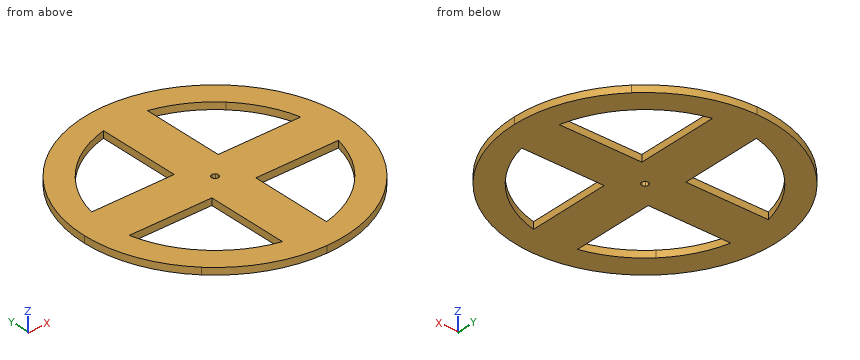
from build123d import *

# Parameters (mm, degrees)
F1_DEPTH = 3.175


with BuildPart() as f1:
    # F0 (on Top) → F1 (new body)
    with BuildSketch(Plane.XY):
        with BuildLine():
            Line((34.677494, 34.677494), (42.656217, 42.656217))
            ThreePointArc((42.656217, 42.656217), (23.085378, 55.733033), (0, 60.325))
            Line((0, 60.325), (0, 48.26))
            Line((0, 48.26), (10.16, 48.26))
            ThreePointArc((10.16, 48.26), (23.374034, 43.193116), (34.677494, 34.677494))
        make_face()
        with BuildLine():
            Line((48.26, 0), (60.325, 0))
            ThreePointArc((60.325, 0), (55.733033, 23.085378), (42.656217, 42.656217))
            Line((42.656217, 42.656217), (34.677494, 34.677494))
            ThreePointArc((34.677494, 34.677494), (43.193116, 23.374034), (48.26, 10.16))
            Line((48.26, 10.16), (48.26, 0))
        make_face()
        with BuildLine():
            Line((0, 48.26), (0, 60.325))
            ThreePointArc((0, 60.325), (-23.085378, 55.733033), (-42.656217, 42.656217))
            Line((-42.656217, 42.656217), (-34.677494, 34.677494))
            ThreePointArc((-34.677494, 34.677494), (-23.374034, 43.193116), (-10.16, 48.26))
            Line((-10.16, 48.26), (0, 48.26))
        make_face()
        with BuildLine():
            Line((-34.677494, 34.677494), (-42.656217, 42.656217))
            ThreePointArc((-42.656217, 42.656217), (-55.733033, 23.085378), (-60.325, 0))
            Line((-60.325, 0), (-48.26, 0))
            Line((-48.26, 0), (-48.26, 10.16))
            ThreePointArc((-48.26, 10.16), (-43.193116, 23.374034), (-34.677494, 34.677494))
        make_face()
        with BuildLine():
            Line((0, 17.78), (0, 48.26))
            Line((0, 48.26), (-10.16, 48.26))
            Line((-10.16, 48.26), (-10.16, 14.591189))
            ThreePointArc((-10.16, 14.591189), (-5.324334, 16.964076), (0, 17.78))
        make_face()
        with BuildLine():
            Line((10.16, 48.26), (0, 48.26))
            Line((0, 48.26), (0, 17.78))
            ThreePointArc((0, 17.78), (5.324334, 16.964076), (10.16, 14.591189))
            Line((10.16, 14.591189), (10.16, 48.26))
        make_face()
        with BuildLine():
            ThreePointArc((10.16, 14.591189), (5.324334, 16.964076), (0, 17.78))
            Line((0, 17.78), (0, 10.16))
            Line((0, 10.16), (10.16, 10.16))
            Line((10.16, 10.16), (10.16, 14.591189))
        make_face()
        with BuildLine():
            Line((0, 10.16), (0, 17.78))
            ThreePointArc((0, 17.78), (-5.324334, 16.964076), (-10.16, 14.591189))
            Line((-10.16, 14.591189), (-10.16, 10.16))
            Line((-10.16, 10.16), (0, 10.16))
        make_face()
        with BuildLine():
            Line((0, 1.5875), (0, 10.16))
            Line((0, 10.16), (-10.16, 10.16))
            Line((-10.16, 10.16), (-1.122532, 1.122532))
            ThreePointArc((-1.122532, 1.122532), (-0.60751, 1.466659), (0, 1.5875))
        make_face()
        with BuildLine():
            Line((-1.122532, 1.122532), (-10.16, 10.16))
            Line((-10.16, 10.16), (-10.16, 0))
            Line((-10.16, 0), (-1.5875, 0))
            ThreePointArc((-1.5875, 0), (-1.466659, 0.60751), (-1.122532, 1.122532))
        make_face()
        with BuildLine():
            ThreePointArc((-14.591189, 10.16), (-16.964076, 5.324334), (-17.78, 0))
            Line((-17.78, 0), (-10.16, 0))
            Line((-10.16, 0), (-10.16, 10.16))
            Line((-10.16, 10.16), (-14.591189, 10.16))
        make_face()
        with BuildLine():
            Line((10.16, 0), (17.78, 0))
            ThreePointArc((17.78, 0), (16.964076, 5.324334), (14.591189, 10.16))
            Line((14.591189, 10.16), (10.16, 10.16))
            Line((10.16, 10.16), (10.16, 0))
        make_face()
        with BuildLine():
            Line((1.122532, 1.122532), (10.16, 10.16))
            Line((10.16, 10.16), (0, 10.16))
            Line((0, 10.16), (0, 1.5875))
            ThreePointArc((0, 1.5875), (0.60751, 1.466659), (1.122532, 1.122532))
        make_face()
        with BuildLine():
            Line((1.5875, 0), (10.16, 0))
            Line((10.16, 0), (10.16, 10.16))
            Line((10.16, 10.16), (1.122532, 1.122532))
            ThreePointArc((1.122532, 1.122532), (1.466659, 0.60751), (1.5875, 0))
        make_face()
        with BuildLine():
            Line((-10.16, 0), (-17.78, 0))
            ThreePointArc((-17.78, 0), (-16.964076, -5.324334), (-14.591189, -10.16))
            Line((-14.591189, -10.16), (-10.16, -10.16))
            Line((-10.16, -10.16), (-10.16, 0))
        make_face()
        with BuildLine():
            Line((-10.16, -10.16), (0, -10.16))
            Line((0, -10.16), (0, -1.5875))
            ThreePointArc((0, -1.5875), (-0.60751, -1.466659), (-1.122532, -1.122532))
            Line((-1.122532, -1.122532), (-10.16, -10.16))
        make_face()
        with BuildLine():
            ThreePointArc((-10.16, -14.591189), (-5.324334, -16.964076), (0, -17.78))
            Line((0, -17.78), (0, -10.16))
            Line((0, -10.16), (-10.16, -10.16))
            Line((-10.16, -10.16), (-10.16, -14.591189))
        make_face()
        with BuildLine():
            Line((0, -10.16), (0, -17.78))
            ThreePointArc((0, -17.78), (5.324334, -16.964076), (10.16, -14.591189))
            Line((10.16, -14.591189), (10.16, -10.16))
            Line((10.16, -10.16), (0, -10.16))
        make_face()
        with BuildLine():
            Line((0, -10.16), (10.16, -10.16))
            Line((10.16, -10.16), (1.122532, -1.122532))
            ThreePointArc((1.122532, -1.122532), (0.60751, -1.466659), (0, -1.5875))
            Line((0, -1.5875), (0, -10.16))
        make_face()
        with BuildLine():
            ThreePointArc((14.591189, -10.16), (16.964076, -5.324334), (17.78, 0))
            Line((17.78, 0), (10.16, 0))
            Line((10.16, 0), (10.16, -10.16))
            Line((10.16, -10.16), (14.591189, -10.16))
        make_face()
        with BuildLine():
            Line((17.78, 0), (48.26, 0))
            Line((48.26, 0), (48.26, 10.16))
            Line((48.26, 10.16), (14.591189, 10.16))
            ThreePointArc((14.591189, 10.16), (16.964076, 5.324334), (17.78, 0))
        make_face()
        with BuildLine():
            Line((48.26, -10.16), (48.26, 0))
            Line((48.26, 0), (17.78, 0))
            ThreePointArc((17.78, 0), (16.964076, -5.324334), (14.591189, -10.16))
            Line((14.591189, -10.16), (48.26, -10.16))
        make_face()
        with BuildLine():
            Line((-48.26, 10.16), (-48.26, 0))
            Line((-48.26, 0), (-17.78, 0))
            ThreePointArc((-17.78, 0), (-16.964076, 5.324334), (-14.591189, 10.16))
            Line((-14.591189, 10.16), (-48.26, 10.16))
        make_face()
        with BuildLine():
            Line((-17.78, 0), (-48.26, 0))
            Line((-48.26, 0), (-48.26, -10.16))
            Line((-48.26, -10.16), (-14.591189, -10.16))
            ThreePointArc((-14.591189, -10.16), (-16.964076, -5.324334), (-17.78, 0))
        make_face()
        with BuildLine():
            Line((-10.16, -48.26), (0, -48.26))
            Line((0, -48.26), (0, -17.78))
            ThreePointArc((0, -17.78), (-5.324334, -16.964076), (-10.16, -14.591189))
            Line((-10.16, -14.591189), (-10.16, -48.26))
        make_face()
        with BuildLine():
            Line((0, -17.78), (0, -48.26))
            Line((0, -48.26), (10.16, -48.26))
            Line((10.16, -48.26), (10.16, -14.591189))
            ThreePointArc((10.16, -14.591189), (5.324334, -16.964076), (0, -17.78))
        make_face()
        with BuildLine():
            ThreePointArc((42.656217, -42.656217), (55.733033, -23.085378), (60.325, 0))
            Line((60.325, 0), (48.26, 0))
            Line((48.26, 0), (48.26, -10.16))
            ThreePointArc((48.26, -10.16), (43.193116, -23.374034), (34.677494, -34.677494))
            Line((34.677494, -34.677494), (42.656217, -42.656217))
        make_face()
        with BuildLine():
            ThreePointArc((0, -60.325), (23.085378, -55.733033), (42.656217, -42.656217))
            Line((42.656217, -42.656217), (34.677494, -34.677494))
            ThreePointArc((34.677494, -34.677494), (23.374034, -43.193116), (10.16, -48.26))
            Line((10.16, -48.26), (0, -48.26))
            Line((0, -48.26), (0, -60.325))
        make_face()
        with BuildLine():
            ThreePointArc((-42.656217, -42.656217), (-23.085378, -55.733033), (0, -60.325))
            Line((0, -60.325), (0, -48.26))
            Line((0, -48.26), (-10.16, -48.26))
            ThreePointArc((-10.16, -48.26), (-23.374034, -43.193116), (-34.677494, -34.677494))
            Line((-34.677494, -34.677494), (-42.656217, -42.656217))
        make_face()
        with BuildLine():
            ThreePointArc((-60.325, 0), (-55.733033, -23.085378), (-42.656217, -42.656217))
            Line((-42.656217, -42.656217), (-34.677494, -34.677494))
            ThreePointArc((-34.677494, -34.677494), (-43.193116, -23.374034), (-48.26, -10.16))
            Line((-48.26, -10.16), (-48.26, 0))
            Line((-48.26, 0), (-60.325, 0))
        make_face()
        with BuildLine():
            Line((10.16, -10.16), (10.16, 0))
            Line((10.16, 0), (1.5875, 0))
            ThreePointArc((1.5875, 0), (1.466659, -0.60751), (1.122532, -1.122532))
            Line((1.122532, -1.122532), (10.16, -10.16))
        make_face()
        with BuildLine():
            Line((-10.16, 0), (-10.16, -10.16))
            Line((-10.16, -10.16), (-1.122532, -1.122532))
            ThreePointArc((-1.122532, -1.122532), (-1.466659, -0.60751), (-1.5875, 0))
            Line((-1.5875, 0), (-10.16, 0))
        make_face()
    extrude(amount=F1_DEPTH)


solid = f1.part
The listing builds one solid part. Answer for the finished solid, in the listing's coordinates (mm). Coordinates: 2 decimals unless noted, no trailing zeros. Loops run counter-clockwise (first coordinate to the right, second up) from the corner with the lowest first, then second, coordinate; pieces in that order, holes last. Notation, with made-up numbers: (8.25, 78) -> (13.25, 78) arc R28 cw to (13.25, 112) -> close; hole circle Ø7 at (15, -27). An arc over 180 degrees is marked (long way). Answer in a Markdown table with one row per item. Add a question column.
1. Consider line 1 (Y direction, x = 23, z = 2); line 2 (Y direction, x = -42, z = 0.6); line 3 (X direction, y = -28.5, z = 0.7). Determine where each line is inside the solid, lowest interval first. Write a range as [from, to].
2. The part is cut by section A-A, the plane z = 1.85. Count the separate pieces of the cut face and the enclosed holes in it, then the cut area to 3 significant figures.
3. The part is cut by section C-C, the plane y = -18. Write down the section's boundary in (x, z) (3 decimals).
4. The part is cut by section B-B, the plane x = 24. Write down the section's boundary in (y, z) (3 decimals), then the cut area to 3 significant figures.
5. Flat-ended cylindrical pins translate along their axes: P1, Ø1.6, axis at y = -32.5, z = 2, coming from the +X side; P2, Ø1, axis at y = 21, z = 1, coming from the -X side; P3, Ø1, axis at y = 35, z = 2, coming from the +X side; P4, Ø6, axis at x = -13.5, y = 2, coming from the -Z side. Find the tip coordinate at first contact, or state that the pin passes through.
Answer below:
| question | item | result |
|---|---|---|
| 1 | line 1 | [-55.77, -43.4], [-10.16, 10.16], [43.4, 55.77] |
| 1 | line 2 | [-43.3, -25.41], [-10.16, 10.16], [25.41, 43.3] |
| 1 | line 3 | [-53.17, -39.94], [-10.16, 10.16], [39.94, 53.17] |
| 2 | separate pieces | 1 |
| 2 | enclosed holes | 5 |
| 2 | area | 7,390 mm2 |
| 3 | outline | (-57.577, 0) -> (-45.771, 0) -> (-45.771, 3.175) -> (-57.577, 3.175) -> close; (-10.16, 0) -> (10.16, 0) -> (10.16, 3.175) -> (-10.16, 3.175) -> close; (45.771, 0) -> (57.577, 0) -> (57.577, 3.175) -> (45.771, 3.175) -> close |
| 4 | outline | (-55.345, 0) -> (-42.841, 0) -> (-42.841, 3.175) -> (-55.345, 3.175) -> close; (-10.16, 0) -> (10.16, 0) -> (10.16, 3.175) -> (-10.16, 3.175) -> close; (42.841, 0) -> (55.345, 0) -> (55.345, 3.175) -> (42.841, 3.175) -> close |
| 4 | area | 144 mm2 |
| 5 | P1 | x = 51.32 |
| 5 | P2 | x = -56.73 |
| 5 | P3 | x = 49.49 |
| 5 | P4 | z = 0 |
